```python
from build123d import *

# Parameters (mm, degrees)
SKETCH1_W               = 25.4
SKETCH1_H               = 25.4
SKETCH1_W_2             = 5.969
SKETCH1_H_2             = 5.969
BOSS_EXTRUDE1_DEPTH     = 10.16
SKETCH2_W               = 1.905
SKETCH2_H               = 9.7155
BOSS_EXTRUDE2_DEPTH     = 1.016
SKETCH3_W               = 9.4488
SKETCH3_H               = 9.4488
SKETCH3_W_2             = 5.969
SKETCH3_H_2             = 5.969
BOSS_EXTRUDE3_DEPTH     = 6
CUT_EXTRUDE2_REACH      = 22.635
SKETCH4_W               = 1.905
SKETCH4_H               = 4.1656
SKETCH7_R               = 1.237436867
CUT_EXTRUDE5_DEPTH      = 25.160413904
MIRROR4_COPY_1_SKETCH_R = 1.237436867
MIRROR4_COPY_1_DEPTH    = 25.160413904
SKETCH6_W               = 25.4
SKETCH6_H               = 25.4
CUT_EXTRUDE4_DEPTH      = 7.62
FILLET1_R               = 1.778


with BuildPart() as part:
    # Sketch1 → Boss-Extrude1 (new body)
    with BuildSketch(Plane(origin=(0, 0, 0), x_dir=(1, 0, 0), z_dir=(0, 1, 0))):
        Rectangle(SKETCH1_W, SKETCH1_H)
        Rectangle(SKETCH1_W_2, SKETCH1_H_2, mode=Mode.SUBTRACT)
    extrude(amount=BOSS_EXTRUDE1_DEPTH)

    # Sketch2 → Boss-Extrude2 (add)
    with BuildSketch(Plane.XZ):
        with Locations((0, 7.84225)):
            Rectangle(SKETCH2_W, SKETCH2_H)
    boss_extrude2 = extrude(amount=BOSS_EXTRUDE2_DEPTH)

    # Mirror1: Boss-Extrude2 across plane
    add(boss_extrude2.mirror(Plane.XY))

    # Sketch3 → Boss-Extrude3 (add)
    with BuildSketch(Plane.XZ):
        Rectangle(SKETCH3_W, SKETCH3_H)
        Rectangle(SKETCH3_W_2, SKETCH3_H_2, mode=Mode.SUBTRACT)
    extrude(amount=BOSS_EXTRUDE3_DEPTH)

    # Sketch4 → Cut-Extrude2 (cut, up to next)
    with BuildSketch(Plane.XZ, mode=Mode.PRIVATE) as cut_extrude2_sk1:
        with Locations((0, 6.8072)):
            Rectangle(SKETCH4_W, SKETCH4_H)
    cut_extrude2_tool1 = extrude(cut_extrude2_sk1.sketch, amount=CUT_EXTRUDE2_REACH, mode=Mode.PRIVATE) & part.part
    # Sketch4 → Cut-Extrude2 (cut, up to next)
    with BuildSketch(Plane.XZ, mode=Mode.PRIVATE) as cut_extrude2_sk2:
        with Locations((0, -6.8072)):
            Rectangle(SKETCH4_W, SKETCH4_H)
    cut_extrude2_tool2 = extrude(cut_extrude2_sk2.sketch, amount=CUT_EXTRUDE2_REACH, mode=Mode.PRIVATE) & part.part
    add(cut_extrude2_tool1.solids().sort_by_distance((0, 0, 6.8072))[0], mode=Mode.SUBTRACT)
    add(cut_extrude2_tool2.solids().sort_by_distance((0, 0, -6.8072))[0], mode=Mode.SUBTRACT)

    # Sketch7 → Cut-Extrude5 (cut, through all)
    with BuildSketch(Plane.XZ.offset(6)):
        with Locations((-2.1095, 2.1095)):
            Circle(SKETCH7_R)
    cut_extrude5 = extrude(amount=-CUT_EXTRUDE5_DEPTH, mode=Mode.SUBTRACT)

    # Mirror3: Cut-Extrude5 across plane
    add(cut_extrude5.mirror(Plane(origin=(0, 0, 0), x_dir=(0, 0, 1), z_dir=(1, 0, 0))), mode=Mode.SUBTRACT)

    # Mirror4: Cut-Extrude5 across plane
    add(cut_extrude5.mirror(Plane.XY), mode=Mode.SUBTRACT)

    # Mirror4 copy 1 sketch → Mirror4 copy 1 (cut, through all)
    with BuildSketch(Plane(origin=(0, -6, 0), x_dir=(-1, 0, 0), z_dir=(0, -1, 0))):
        with Locations((-2.1095, 2.1095)):
            Circle(MIRROR4_COPY_1_SKETCH_R)
    extrude(amount=-MIRROR4_COPY_1_DEPTH, mode=Mode.SUBTRACT)

    # Sketch6 → Cut-Extrude4 (cut)
    with BuildSketch(Plane(origin=(0, 10.16, 0), x_dir=(1, 0, 0), z_dir=(0, 1, 0))):
        Rectangle(SKETCH6_W, SKETCH6_H)
    extrude(amount=-CUT_EXTRUDE4_DEPTH, mode=Mode.SUBTRACT)

    # Fillet1
    fillet1_edges = [part.edges().sort_by_distance(p)[0] for p in [
        (4.7244, -3, 4.7244),
        (-4.7244, -3, 4.7244),
        (-4.7244, -3, -4.7244),
        (4.7244, -3, -4.7244),
    ]]
    fillet(fillet1_edges, radius=FILLET1_R)


solid = part.part
```
Design review of the part built by this model. Coordinates are the model's own, in mm. A direction names the side the tool comes from. Coordinates: 2 decimals unless noted, no trailing zeros. Loops run counter-clockwise (first coordinate to the right, second up) from the corner with the lowest first, then second, coordinate; pieces in that order, holes last. Notation, with made-up numbers: (65.5, 81.25) - (117.5, 81.25) arc R9 ccw to (117.5, 97.25) - close; hole circle Ø9 at (58, -4.5). An arc over 180 degrees is marked (long way). Use CSV: the item, a comma, the result in double quotes. Start each with the question number.
1) For pin 1 Ø1.5 at (x, z) = (0.5, -11.5) entering from -Y; pin 2 Ø3 at (x, y) = (0, -3.5) entering from +Z; pin 3 Ø0.5 at (y, z) = (-0.5, 10) entering from +X; pin 4 Ø1.1 at (y, z) = (-0.5, -11.5) entering from +X, all flat-tipped, find the tip position at first contact; note any pin that passes through.
2) Tool access review of faces 5 (the flat face through (2.984, -2, 0)), 6 (the flat face through (0.952, -0.5, -10.8)), 7 (the flat face through (-0.952, -0.5, 10.8)), 8 (the cylindrical face through (-4.217, -3.042, -4.19)), 9 (the flat face through (0, -0.5, 8.89)): name each direction out of +Z, -Z, +X, -X, +Y, -Y from which nothing blocks a thin tool from reaching the whole face with its end or side.
3) Consider section C-C on x = 0. Write out the cut boundary in (y, z).
4) The part is to be moulded in two halves that separate along Z. For faces 1 (the cylindrical face through (4.19, -3.042, -4.217)), 2 (the cylindrical face through (2.97, -1.79, 3)), 3 (the cylindrical face through (-2.97, -1.79, 3)), 4 (the flat face through (4.724, -3, 0)), say which applies: +Z half, -Z half, draft (parallel to the pull), parting line (faces both ways), or undercut.
5) Consider section D-D on x = 3.75. Write out the cut boundary in (y, z).
6) Wall thickness on L1, parallel to X at y = -3.5, z = 2; L2, parallel to X at y = 2.25, z = -0.75; L3, parallel to Y at x = -9, z = -7.25: over which ranges is each line inside the solid? List them lowest first. Write a range as from..to.
7) Consider section B-B on y = -1.5. Write out the cut boundary in (x, z).
8) Consider section A-A on z = 0. Write out the cut boundary in (x, y).
Geometry says:
1,pin 1,"y = -1.02"
1,pin 2,"z = 4.72"
1,pin 3,"x = 0.95"
1,pin 4,"x = 12.7"
2,face 5,"+Y, -Y"
2,face 6,"-Z, +X, -Y"
2,face 7,"+Z, -X, -Y"
2,face 8,"-Z, -X, -Y"
2,face 9,"+X, -X, -Y"
3,outline,"(-6, -4.72) - (0, -4.72) - (0, -8.89) - (-1.02, -8.89) - (-1.02, -12.7) - (2.54, -12.7) - (2.54, -2.98) - (-6, -2.98) - close; (-6, 2.98) - (2.54, 2.98) - (2.54, 12.7) - (-1.02, 12.7) - (-1.02, 8.89) - (0, 8.89) - (0, 4.72) - (-6, 4.72) - close"
4,face 1,"-Z half"
4,face 2,"undercut"
4,face 3,"undercut"
4,face 4,"draft"
5,outline,"(-6, -4.53) - (0, -4.53) - (0, -12.7) - (2.54, -12.7) - (2.54, 12.7) - (0, 12.7) - (0, 4.53) - (-6, 4.53) - close"
6,L1,"-4.72..-3.34, 3.34..4.72"
6,L2,"-12.7..-2.98, 2.98..12.7"
6,L3,"0..2.54"
7,outline,"(-4.72, -2.95) arc R1.78 ccw to (-2.95, -4.72) - (2.95, -4.72) arc R1.78 ccw to (4.72, -2.95) - (4.72, 2.95) arc R1.78 ccw to (2.95, 4.72) - (-2.95, 4.72) arc R1.78 ccw to (-4.72, 2.95) - close; hole (-2.98, -1.23) arc R1.24 ccw to (-1.23, -2.98) - (1.23, -2.98) arc R1.24 ccw to (2.98, -1.23) - (2.98, 1.23) arc R1.24 ccw to (1.23, 2.98) - (-1.23, 2.98) arc R1.24 ccw to (-2.98, 1.23) - close"
8,outline,"(-12.7, 0) - (-4.72, 0) - (-4.72, -6) - (-2.98, -6) - (-2.98, 2.54) - (-12.7, 2.54) - close; (2.98, -6) - (4.72, -6) - (4.72, 0) - (12.7, 0) - (12.7, 2.54) - (2.98, 2.54) - close"
